```python
from build123d import *

# Parameters (mm, degrees)
CUT_EXTRUDE1_REACH      = 17.5
SKETCH2_R               = 1.75
SKETCH3_W               = 4
SKETCH3_H               = 4
CUT_EXTRUDE2_DEPTH      = 12
CUT_EXTRUDE2_DEPTH_BACK = 12


with BuildPart() as part:
    # Sketch1 → Revolve1 (revolve)
    with BuildSketch(Plane(origin=(0, 0, 0), x_dir=(1, 0, 0), z_dir=(0, 1, 0))):
        Polygon((-15.5, 4), (-15.5, 5.25), (-4, 5.25), (-4, 11), (0, 11), (0, 4), align=None)
    revolve(axis=Axis((-43.707317073, 0, 0), (1, 0, 0)))

    # Sketch2 → Cut-Extrude1 (cut, up to next)
    with BuildSketch(Plane(origin=(0, 0, 0), x_dir=(0, 0, -1), z_dir=(1, 0, 0)), mode=Mode.PRIVATE) as cut_extrude1_sk1:
        with Locations((0, 8)):
            Circle(SKETCH2_R)
    cut_extrude1_tool1 = extrude(cut_extrude1_sk1.sketch, amount=-CUT_EXTRUDE1_REACH, mode=Mode.PRIVATE) & part.part
    add(cut_extrude1_tool1.solids().sort_by_distance((0, 8, 0))[0], mode=Mode.SUBTRACT)
    # Sketch2 → Cut-Extrude1 (cut, up to next)
    with BuildSketch(Plane(origin=(0, 0, 0), x_dir=(0, 0, -1), z_dir=(1, 0, 0)), mode=Mode.PRIVATE) as cut_extrude1_sk2:
        with Locations((8, 0)):
            Circle(SKETCH2_R)
    cut_extrude1_tool2 = extrude(cut_extrude1_sk2.sketch, amount=-CUT_EXTRUDE1_REACH, mode=Mode.PRIVATE) & part.part
    add(cut_extrude1_tool2.solids().sort_by_distance((0, 0, -8))[0], mode=Mode.SUBTRACT)
    # Sketch2 → Cut-Extrude1 (cut, up to next)
    with BuildSketch(Plane(origin=(0, 0, 0), x_dir=(0, 0, -1), z_dir=(1, 0, 0)), mode=Mode.PRIVATE) as cut_extrude1_sk3:
        with Locations((0, -8)):
            Circle(SKETCH2_R)
    cut_extrude1_tool3 = extrude(cut_extrude1_sk3.sketch, amount=-CUT_EXTRUDE1_REACH, mode=Mode.PRIVATE) & part.part
    add(cut_extrude1_tool3.solids().sort_by_distance((0, -8, 0))[0], mode=Mode.SUBTRACT)
    # Sketch2 → Cut-Extrude1 (cut, up to next)
    with BuildSketch(Plane(origin=(0, 0, 0), x_dir=(0, 0, -1), z_dir=(1, 0, 0)), mode=Mode.PRIVATE) as cut_extrude1_sk4:
        with Locations((-8, 0)):
            Circle(SKETCH2_R)
    cut_extrude1_tool4 = extrude(cut_extrude1_sk4.sketch, amount=-CUT_EXTRUDE1_REACH, mode=Mode.PRIVATE) & part.part
    add(cut_extrude1_tool4.solids().sort_by_distance((0, 0, 8))[0], mode=Mode.SUBTRACT)

    # Sketch3 → Cut-Extrude2 (cut, two sides)
    with BuildSketch(Plane.XY) as cut_extrude2_sk:
        with Locations((-13.5, 0)):
            Rectangle(SKETCH3_W, SKETCH3_H)
    extrude(amount=CUT_EXTRUDE2_DEPTH, mode=Mode.SUBTRACT)
    extrude(cut_extrude2_sk.sketch, amount=-CUT_EXTRUDE2_DEPTH_BACK, mode=Mode.SUBTRACT)


solid = part.part
```
For this review, take the finished solid that the model builds, in its own axes (mm). A direction names the side the tool comes from. Round coordinates to 2 decimals unless told otherwise and drop trailing zeros. Write each loop counter-clockwise with the first axis right and the second up, starting at its lowest first coordinate (ties: lowest second). Pieces come first, ordered by that corner, then holes. Notation, with made-up numbers: (-21, 15.25) -> (36, 15.25) arc R18 cw to (36, 47.25) -> close; hole circle Ø8 at (-5.75, -40). An arc over 180 degrees is marked (long way). Use one line per item in the form item = value.
1) Clearance check with flat-ended pins moving along their axes: pin 1 (1.5 mm diameter, centred on x = -10, z = 4.5, fed in from -Y); pin 2 (4.5 mm diameter, centred on y = 0, z = -8, fed in from -X); pin 3 (4 mm diameter, centred on x = -5, y = 2.5, fed in from +Z); pin 4 (2 mm diameter, centred on y = -8, z = 0, fed in from +X). State where each tip first meets the part, or that it passes through.
Found:
pin_1 = -3.67
pin_2 = -4
pin_3 = 10.97
pin_4 = through
2) Take a section at B-B, the plane z = 0. Write out the cut boundary in (x, y).
Found:
outline = (-15.5, -5.25) -> (-4, -5.25) -> (-4, -6.25) -> (0, -6.25) -> (0, -4) -> (-15.5, -4) -> close; (-15.5, 4) -> (0, 4) -> (0, 6.25) -> (-4, 6.25) -> (-4, 5.25) -> (-15.5, 5.25) -> close; (-4, -11) -> (0, -11) -> (0, -9.75) -> (-4, -9.75) -> close; (-4, 9.75) -> (0, 9.75) -> (0, 11) -> (-4, 11) -> close
3) Mouldability with a two-part tool opening along Y and no side actions: class faces 4 (the flat face through (-15.5, 4.4, -0.1)), 5 (the cylindrical face through (-1.972, 0.526, -9.669)), 6 (the cylindrical face through (-9.67, -4.66, -2.42)) as +Y half, -Y half, draft (parallel to the pull), parting line (faces both ways), or undercut.
Found:
face_4 = draft
face_5 = undercut
face_6 = parting line
4) To check wall thickness, follow L1, parallel to Y at x = -11.75, z = 0; L2, parallel to Y at x = -3.1, z = 0; L3, parallel to Z at x = -2.5, y = 1.5. State the ranges of each line that lie inside material, in increasing order. Write a range as from..to.
Found:
L1 = -5.25..-4, 4..5.25
L2 = -11..-9.75, -6.25..-4, 4..6.25, 9.75..11
L3 = -10.9..-8.9, -7.1..-3.71, 3.71..7.1, 8.9..10.9
5) Take a section at C-C, the plane y = 0. Write out the cut boundary in (x, z), and give its area (4 significant figures).
Found:
outline = (-11.5, -5.25) -> (-4, -5.25) -> (-4, -6.25) -> (0, -6.25) -> (0, -4) -> (-11.5, -4) -> close; (-11.5, 4) -> (0, 4) -> (0, 6.25) -> (-4, 6.25) -> (-4, 5.25) -> (-11.5, 5.25) -> close; (-4, -11) -> (0, -11) -> (0, -9.75) -> (-4, -9.75) -> close; (-4, 9.75) -> (0, 9.75) -> (0, 11) -> (-4, 11) -> close
area = 46.75 mm2
6) Take a section at D-D, the plane x = -0.75. Write out the cut boundary in (y, z), and give its area (3 significant figures).
Found:
outline = circle Ø22 at (0, 0); hole circle Ø3.5 at (-8, 0); hole circle Ø8 at (0, 0); hole circle Ø3.5 at (0, -8); hole circle Ø3.5 at (0, 8); hole circle Ø3.5 at (8, 0)
area = 291 mm2
7) Take a section at A-A, the plane x = -13. Write out the cut boundary in (y, z), and give its area (3 significant figures).
Found:
outline = (-2, -4.85) -> (-2, -3.46) arc R4 cw to (-2, 3.46) -> (-2, 4.85) arc R5.25 ccw to start; (2, -4.85) arc R5.25 ccw to (2, 4.85) -> (2, 3.46) arc R4 cw to (2, -3.46) -> close
area = 26.0 mm2
8) Tool access review of faces 1 (the flat face through (0, 0, -5)), 2 (the flat face through (-4, 3, 5)), 3 (the flat face through (-14, 2, 4)): name each direction out of +Z, -Z, +X, -X, +Y, -Y from which nothing blocks a thin tool from reaching the whole face with its end or side.
Found:
face_1 = +Z, -Z, +X, +Y, -Y
face_2 = -X
face_3 = +Z, -Z, -X
